from build123d import *

# Parameters (mm, degrees)
SKETCH1_R           = 44.45
SKETCH1_R_2         = 2.921
BOSS_EXTRUDE1_DEPTH = 12.7
SKETCH2_R           = 12.7
BOSS_EXTRUDE2_DEPTH = 127
CUT_EXTRUDE1_REACH  = 159.347
SKETCH4_R           = 2.921


with BuildPart() as part:
    # Sketch1 → Boss-Extrude1 (new body)
    with BuildSketch(Plane.XY):
        Circle(SKETCH1_R)
        with Locations((0, 20.32)):
            Circle(SKETCH1_R_2, mode=Mode.SUBTRACT)
        with Locations((19.325468411, 6.279225326)):
            Circle(SKETCH1_R_2, mode=Mode.SUBTRACT)
        with Locations((11.943796327, -16.439225326)):
            Circle(SKETCH1_R_2, mode=Mode.SUBTRACT)
        with Locations((-11.943796327, -16.439225326)):
            Circle(SKETCH1_R_2, mode=Mode.SUBTRACT)
        with Locations((-19.325468411, 6.279225326)):
            Circle(SKETCH1_R_2, mode=Mode.SUBTRACT)
    extrude(amount=BOSS_EXTRUDE1_DEPTH)

    # Sketch2 → Boss-Extrude2 (add)
    with BuildSketch(Plane.XY.offset(12.7)):
        Circle(SKETCH2_R)
    extrude(amount=BOSS_EXTRUDE2_DEPTH)

    # Sketch4 → Cut-Extrude1 (cut, up to next)
    with BuildSketch(Plane(origin=(0, -12.7, 0), x_dir=(-1, 0, 0), z_dir=(0, -1, 0)), mode=Mode.PRIVATE) as cut_extrude1_sk1:
        with Locations(Location((0, -133.35, 0), (0, 0, 90))):
            Circle(SKETCH4_R)
    cut_extrude1_tool1 = extrude(cut_extrude1_sk1.sketch, amount=-CUT_EXTRUDE1_REACH, mode=Mode.PRIVATE) & part.part
    add(cut_extrude1_tool1.solids().sort_by_distance((0, -12.7, 133.35))[0], mode=Mode.SUBTRACT)


solid = part.part
Could you check a few things on this model? Use its own coordinates, in mm. A direction names the side the tool comes from. Give positions to 0.01 mm unless a question says otherwise; leave off trailing zeros. Write each loop counter-clockwise with the first axis right and the second up, starting at its lowest first coordinate (ties: lowest second). Pieces come first, ordered by that corner, then holes. Notation, with made-up numbers: (53, 24) -> (92, 24) arc R33 ccw to (92, 62) -> close; hole circle Ø1 at (29, -28.5). An arc over 180 degrees is marked (long way). Answer as CSV lines item,"result". Start each with the question number.
(1) Please list where these lines run through material, in increasing order: line 1 (Z direction, x = 0, y = -2); line 2 (Y direction, x = 0, z = 8); line 3 (X direction, y = -0.5, z = 133.35).
(2) If we section it at B-B, the plane y = 20.32: Write out the boundary of the cut face in (x, z), and give its area (3 significant figures).
(3) If we section it at D-D, the plane x = 11: Write out the boundary of the cut face in (y, z).
(4) If we mould it in two halves opening along Y, with no side actions, what happens to faces 3 (the face through (9.3, -9.3, 12.7)), 4 (the face through (22.11, 7.16, 6.26)), 5 (the face through (42.397, 13.352, 6.261))? For each: +Y half, -Y half, draft (parallel to the pull), parting line (faces both ways), or undercut.
(5) Which directions (+Z, -Z, +X, -X, +Y, -Y) give clear straight access to the entire face, cutting with the end or side of a thin tool? Please do faces 1 (the face through (-2.75, -12.4, 75.31)), 2 (the face through (-12.58, -19.29, 6.26)).
(6) I'm going to push flat-ended pins straight in: pin 1 Ø6.5 at (x, y) = (-19.33, 6.28) entering from +Z; pin 2 Ø12 at (y, z) = (12, 107.5) entering from -X; pin 3 Ø4.5 at (x, y) = (11.94, -16.44) entering from +Z; pin 4 Ø7.5 at (x, y) = (-11.94, -16.44) entering from -Z. Where does each tip first touch, or does it pass through?
(7) If we section it at C-C, the plane y = 0: Write out the boundary of the cut face in (x, z).
(8) If we section it at A-A, the plane x = 0: Write out the boundary of the cut face in (y, z).
Answer list:
1,line 1,"0 to 130.43, 136.27 to 139.7"
1,line 2,"-44.45 to 17.4, 23.24 to 44.45"
1,line 3,"-12.69 to -2.92, 2.92 to 12.69"
2,outline,"(-39.53, 0) -> (-2.92, 0) -> (-2.92, 12.7) -> (-39.53, 12.7) -> close; (2.92, 0) -> (39.53, 0) -> (39.53, 12.7) -> (2.92, 12.7) -> close"
2,area,"930 mm^2"
3,outline,"(-43.07, 0) -> (-19.2, 0) -> (-19.2, 12.7) -> (-43.07, 12.7) -> close; (-13.67, 0) -> (43.07, 0) -> (43.07, 12.7) -> (6.35, 12.7) -> (6.35, 139.7) -> (-6.35, 139.7) -> (-6.35, 12.7) -> (-13.67, 12.7) -> close"
4,face 3,"draft"
4,face 4,"undercut"
4,face 5,"parting line"
5,face 1,"+Z"
5,face 2,"+Z, -Z"
6,pin 1,"z = 12.7"
6,pin 2,"x = -11.19"
6,pin 3,"through"
6,pin 4,"z = 0"
7,outline,"(-44.45, 0) -> (44.45, 0) -> (44.45, 12.7) -> (12.7, 12.7) -> (12.7, 139.7) -> (-12.7, 139.7) -> (-12.7, 12.7) -> (-44.45, 12.7) -> close; hole circle Ø5.84 at (0, 133.35)"
8,outline,"(-44.45, 0) -> (17.4, 0) -> (17.4, 12.7) -> (12.7, 12.7) -> (12.7, 130.43) -> (-12.7, 130.43) -> (-12.7, 12.7) -> (-44.45, 12.7) -> close; (-12.7, 136.27) -> (12.7, 136.27) -> (12.7, 139.7) -> (-12.7, 139.7) -> close; (23.24, 0) -> (44.45, 0) -> (44.45, 12.7) -> (23.24, 12.7) -> close"
